```python
from build123d import *

# Parameters (mm, degrees)
SKETCH1_W          = 150
SKETCH1_H          = 225
BASE_FLANGE1_DEPTH = 3
SKETCH6_R          = 2.5
SKETCH6_R_2        = 3
CUT_EXTRUDE1_DEPTH = 10
CUT_EXTRUDE2_DEPTH = 10


# Sheet-metal steps are written as plain solids
with BuildPart() as part:
    # Sketch1 → Base-Flange1 (new body)
    with BuildSketch(Plane.XY):
        Rectangle(SKETCH1_W, SKETCH1_H)
    extrude(amount=BASE_FLANGE1_DEPTH)

    # Sketch6 → Cut-Extrude1 (cut)
    with BuildSketch(Plane.XY.offset(3)):
        with Locations((16, 107.5)):
            Circle(SKETCH6_R)
        with Locations((-16, 107.5)):
            Circle(SKETCH6_R)
        with Locations((-16, 75.5)):
            Circle(SKETCH6_R)
        with Locations((16, 75.5)):
            Circle(SKETCH6_R)
        with Locations((9, 53.5)):
            Circle(SKETCH6_R)
        with Locations(Location((16, 7.5, 0), (0, 0, 180))):
            Circle(SKETCH6_R)
        with Locations(Location((16, -24.5, 0), (0, 0, 180))):
            Circle(SKETCH6_R)
        with Locations(Location((-16, 7.5, 0), (0, 0, 180))):
            Circle(SKETCH6_R)
        with Locations(Location((-16, -24.5, 0), (0, 0, 180))):
            Circle(SKETCH6_R)
        with Locations((65, 91.5)):
            Circle(SKETCH6_R_2)
        with Locations((65, 71.5)):
            Circle(SKETCH6_R_2)
        with Locations((65, 51.5)):
            Circle(SKETCH6_R_2)
        with Locations((65, 31.5)):
            Circle(SKETCH6_R_2)
        with Locations((65, 11.5)):
            Circle(SKETCH6_R_2)
        with Locations((65, -8.5)):
            Circle(SKETCH6_R_2)
        with Locations((65, -28.5)):
            Circle(SKETCH6_R_2)
        with Locations((65, -48.5)):
            Circle(SKETCH6_R_2)
        with Locations(Location((-65, -48.5, 0), (0, 0, 180))):
            Circle(SKETCH6_R_2)
        with Locations(Location((-65, -28.5, 0), (0, 0, 180))):
            Circle(SKETCH6_R_2)
        with Locations(Location((-65, -8.5, 0), (0, 0, 180))):
            Circle(SKETCH6_R_2)
        with Locations(Location((-65, 11.5, 0), (0, 0, 180))):
            Circle(SKETCH6_R_2)
        with Locations(Location((-65, 31.5, 0), (0, 0, 180))):
            Circle(SKETCH6_R_2)
        with Locations(Location((-65, 51.5, 0), (0, 0, 180))):
            Circle(SKETCH6_R_2)
        with Locations(Location((-65, 71.5, 0), (0, 0, 180))):
            Circle(SKETCH6_R_2)
        with Locations(Location((-65, 91.5, 0), (0, 0, 180))):
            Circle(SKETCH6_R_2)
        with Locations(Location((9, 29.5, 0), (0, 0, 180))):
            Circle(SKETCH6_R)
        with Locations((-9, 29.5)):
            Circle(SKETCH6_R)
        with Locations(Location((-9, 53.5, 0), (0, 0, 180))):
            Circle(SKETCH6_R)
        with Locations(Location((-65, -68.5, 0), (0, 0, 180))):
            Circle(SKETCH6_R_2)
        with Locations((65, -68.5)):
            Circle(SKETCH6_R_2)
        with Locations(Location((-65, -88.5, 0), (0, 0, 180))):
            Circle(SKETCH6_R_2)
        with Locations((65, -88.5)):
            Circle(SKETCH6_R_2)
    extrude(amount=-CUT_EXTRUDE1_DEPTH, mode=Mode.SUBTRACT)

    # Sketch7 → Cut-Extrude2 (cut)
    with BuildSketch(Plane.XY.offset(3)):
        with BuildLine():
            Line((-50, -112.5), (50, -112.5))
            Line((50, -112.5), (50, -44.5))
            ThreePointArc((50, -44.5), (47.071067812, -37.428932188), (40, -34.5))
            Line((40, -34.5), (-40, -34.5))
            ThreePointArc((-40, -34.5), (-47.071067812, -37.428932188), (-50, -44.5))
            Line((-50, -44.5), (-50, -112.5))
        make_face()
        with BuildLine():
            Line((-42.5, -11), (-42.5, 89))
            ThreePointArc((-42.5, 89), (-37.5, 94), (-32.5, 89))
            Line((-32.5, 89), (-32.5, -11))
            ThreePointArc((-32.5, -11), (-37.5, -16), (-42.5, -11))
        make_face()
        with BuildLine():
            Line((42.5, -11), (42.5, 89))
            ThreePointArc((42.5, 89), (37.5, 94), (32.5, 89))
            Line((32.5, 89), (32.5, -11))
            ThreePointArc((32.5, -11), (37.5, -16), (42.5, -11))
        make_face()
    extrude(amount=-CUT_EXTRUDE2_DEPTH, mode=Mode.SUBTRACT)


solid = part.part
```
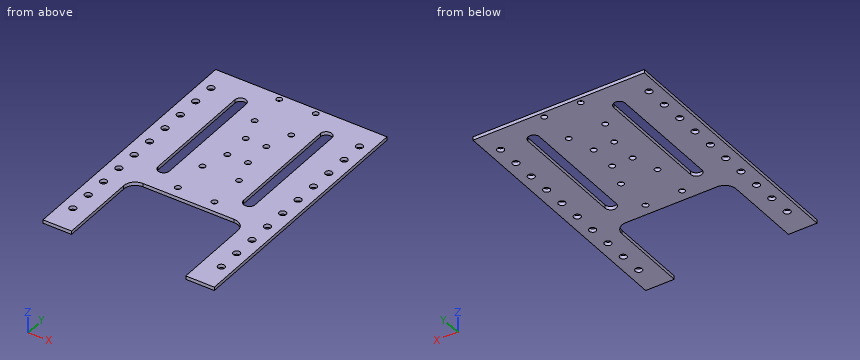
The model under review builds one solid part; all positions refer to its coordinate system, in mm. Round coordinates to 2 decimals unless told otherwise and drop trailing zeros. Order: outer loops, then holes, each group sorted by start corner. A loop starts at its lowest first (then second) coordinate and runs counter-clockwise, first axis right, second up.
(1) Wall thickness on L1, parallel to X at y = 61.5, z = 2.5; L2, parallel to Y at x = 9, z = 2.15; L3, parallel to Y at x = 38, z = 1.25: over which ranges is each line inside the solid? List them lowest first.
Working result:
L1: x = -75 to -42.5, -32.5 to 32.5, 42.5 to 75
L2: y = -34.5 to 27, 32 to 51, 56 to 112.5
L3: y = -34.5 to -15.97, 93.97 to 112.5
(2) Take a section at C-C, the plane y = 107.5. State the section outline as (x, z) points, plus the area to 3 significant figures.
Working result:
outline: (-75, 0) - (-18.5, 0) - (-18.5, 3) - (-75, 3) - close; (-13.5, 0) - (13.5, 0) - (13.5, 3) - (-13.5, 3) - close; (18.5, 0) - (75, 0) - (75, 3) - (18.5, 3) - close
area: 420 mm2
(3) For P1, Ø5, axis at x = 65, y = -88.5, coming from the -Z side, flat-tipped, find the tip position at first contact; note if it passes through.
Working result:
P1: passes through
(4) Take a section at A-A, the plane y = -68.5. State the section outline as (x, z) points, plus the area to 3 significant figures.
Working result:
outline: (-75, 0) - (-68, 0) - (-68, 3) - (-75, 3) - close; (-62, 0) - (-50, 0) - (-50, 3) - (-62, 3) - close; (50, 0) - (62, 0) - (62, 3) - (50, 3) - close; (68, 0) - (75, 0) - (75, 3) - (68, 3) - close
area: 114 mm2
(5) Take a section at B-B, the plane x = -37.5. State the section outline as (y, z) points.
Working result:
outline: (-34.5, 0) - (-16, 0) - (-16, 3) - (-34.5, 3) - close; (94, 0) - (112.5, 0) - (112.5, 3) - (94, 3) - close
(6) Take a section at D-D, the plane x = 9. State the section outline as (y, z) points, plus the area to 3 significant figures.
Working result:
outline: (-34.5, 0) - (27, 0) - (27, 3) - (-34.5, 3) - close; (32, 0) - (51, 0) - (51, 3) - (32, 3) - close; (56, 0) - (112.5, 0) - (112.5, 3) - (56, 3) - close
area: 411 mm2
